Source: CAD feature listing. Evaluate the final solid. Frame: model axes, mm. A direction names the side the tool comes from. Coordinates: 2 decimals unless noted, no trailing zeros. Order: outer loops, then holes, each group sorted by start corner. A loop starts at its lowest first (then second) coordinate and runs counter-clockwise, first axis right, second up. Notation, with made-up numbers: (79, 26.25) - (101, 26.25) arc R25 ccw to (101, 62.25) - close; hole circle Ø2 at (0, 3.25). An arc over 180 degrees is marked (long way). One line per question, with ' | ' between items. Start each with the question number.
(1) Contact query for flat-ended pins moving along their axis: P1, Ø1, axis at x = 1.5, z = -112, coming from the +Y side; P2, Ø4, axis at y = 1.5, z = -59.5, coming from the -X side; P3, Ø1, axis at x = 1.5, z = -177.5, coming from the -Y side; P4, Ø1.5, axis at x = 3, z = 2, coming from the -Y side. Output: stop coordinate, or through.
(2) Line query: line 1 along Z through (x, y) = (3, -0.25); line 2 along Z through (x, y) = (4.15, 1.5); line 3 along Y through (x, z) = (3.3, -212). Output: solid intervals per line, ascending.
(3) Draft query along Z for faces 1 (the cylindrical face through (2.46, 0.51, -226.99)), 2 (the flat face through (0, 0, -108)). Return one class per face: +Z half, -Z half, draft (parallel to the pull), parting line (faces both ways), or undercut.
(4) Section B-B (z = -212). Return the cut outline in (x, y).
(5) Access query for faces 3 (the flat face through (2, 10, -105)), 4 (the flat face through (5, 0, -108)), 5 (the cylindrical face through (2, 0, -8)), 6 (the flat face through (2, -10, -107)). Directions: +Z, -Z, +X, -X, +Y, -Y. A direction counts if a zero-diameter tool reaches every point of the face in a straight line with its end or side. Return the directions, or none.
(6) Section D-D (z = 0). Return the cut outline in (x, y).
(7) Section A-A (y = 0). Return the cut outline in (x, z), then the cut area to 3 significant figures.
(8) Section C-C (x = 3.4). Return the cut outline in (y, z), then the cut area to 3 significant figures.
from build123d import *

# Parameters (mm, degrees)
BOSS_EXTRU_1_DEPTH = 5
TROU_TARAUD_M101_D = 8.5


with BuildPart() as part:
    # Esquisse1 → Boss.-Extru.1 (new body)
    with BuildSketch(Plane(origin=(0, 0, 0), x_dir=(0, 0, -1), z_dir=(1, 0, 0))):
        with BuildLine():
            Line((11.180339887, 10), (200.819660113, 10))
            ThreePointArc((200.819660113, 10), (227, 0), (200.819660113, -10))
            Line((200.819660113, -10), (11.180339887, -10))
            ThreePointArc((11.180339887, -10), (-15, 0), (11.180339887, 10))
        make_face()
        with BuildLine():
            Line((-4.663689527, -6.5), (4.663689527, -6.5))
            ThreePointArc((4.663689527, -6.5), (8, 0), (4.663689527, 6.5))
            Line((4.663689527, 6.5), (-4.663689527, 6.5))
            ThreePointArc((-4.663689527, 6.5), (-8, 0), (-4.663689527, -6.5))
        make_face(mode=Mode.SUBTRACT)
    extrude(amount=BOSS_EXTRU_1_DEPTH)

    # Trou taraudé M101 (through all)
    with Locations(Plane(origin=(5, 0, 0), x_dir=(0, 0, -1), z_dir=(1, 0, 0))):
        with Locations((212, 0)):
            Hole(TROU_TARAUD_M101_D / 2)


solid = part.part
Response values:
1) P1: stops at y = 10 | P2: stops at x = 0 | P3: stops at y = -10 | P4: stops at y = -14.95
2) line 1: z = -227 to -216.24, -207.76 to -8, 8 to 15 | line 2: z = -226.92 to -215.98, -208.02 to -7.86, 7.86 to 14.92 | line 3: y = -15 to -4.25, 4.25 to 15
3) face 1: undercut | face 2: draft
4) outline: (0, -15) - (5, -15) - (5, -4.25) - (0, -4.25) - close; (0, 4.25) - (5, 4.25) - (5, 15) - (0, 15) - close
5) face 3: +X, -X, +Y | face 4: +Z, -Z, +X, +Y, -Y | face 5: +X, -X | face 6: +X, -X, -Y
6) outline: (0, -15) - (5, -15) - (5, -6.5) - (0, -6.5) - close; (0, 6.5) - (5, 6.5) - (5, 15) - (0, 15) - close
7) outline: (0, -227) - (5, -227) - (5, -216.25) - (0, -216.25) - close; (0, -207.75) - (5, -207.75) - (5, -8) - (0, -8) - close; (0, 8) - (5, 8) - (5, 15) - (0, 15) - close | area: 1,090 mm²
8) outline: (-10, -200.82) arc R15 ccw (long way) to (10, -200.82) - (10, -11.18) arc R15 ccw (long way) to (-10, -11.18) - close; hole (-6.5, -4.66) arc R8 ccw to (6.5, -4.66) - (6.5, 4.66) arc R8 ccw to (-6.5, 4.66) - close; hole circle Ø8.5 at (0, -212) | area: 4,860 mm²
